```python
from build123d import *


with BuildPart() as f2:
    # F2: sweep along a path in F1
    with BuildLine(Plane.XY) as f2_path:
        Line((0, 0), (0, 50.8))
        ThreePointArc((0, 50.8), (-20.17757, 70.97757), (-40.35514, 50.8))
    # F0 (on Front) → F2 (sweep)
    with BuildSketch(Plane.XZ):
        Polygon((11.046861, 1.856294), (7.269184, 8.522789), (0.090175, 11.201377), (-7.131028, 8.638716), (-11.015544, 2.033904), (-9.745764, -5.522594), (-3.915833, -10.495009), (3.74636, -10.556693), (9.655589, -5.678782), align=None)
    sweep(path=f2_path.line)


solid = f2.part
```
Check sheet for the modelled part. Datum: model origin and axes. Units: mm. A direction names the side the tool comes from. Give positions to 0.01 mm unless a question says otherwise; leave off trailing zeros. Order: outer loops, then holes, each group sorted by start corner. A loop starts at its lowest first (then second) coordinate and runs counter-clockwise, first axis right, second up. Notation, with made-up numbers: (1, 12.5) -> (23, 12.5) arc R19 ccw to (23, 26.5) -> close; hole circle Ø8 at (50, 1.25). An arc over 180 degrees is marked (long way). Use CSV: the item, a comma, the result in double quotes. Start each with the question number.
1) Sectioned sample at C-C, the plane z = -2.75. Record the boundary of the cut face in (x, y).
2) Set-up check for faces 4 (the face through (-19.64, 75.09, -10.25)), 5 (the face through (-9.046, 25.756, 5.383)), 6 (the face through (9.184, 25.756, 5.143)), 7 (the face through (-41, 50.8, 0)), 8 (the face through (-6.872, 25.756, -7.974)): record each of +Z, -Z, +X, -X, +Y, -Y from which the full face is reachable in a straight line by a thin tool's end or side.
3) Material ranges on line 1 (X direction, y = 55, z = -1.25); line 2 (X direction, y = 53, z = 7); line 3 (Y direction, x = -11, z = 8), recorded low to high. Write a range as from..to.
4) Go/stop test with flat-tipped pins: P1, Ø10, axis at x = -6, y = 32, coming from the -Z side; P2, Ø2, axis at x = -4.5, y = 14, coming from the +Z side; P3, Ø2, axis at x = -28, z = -0.5, coming from the -Y side. Record where each tip stops, or that it passes through.
5) Mould release check, pull along X, two halves, no side actions. Record for faces 1 (the face through (-19.94, 61.59, -5.83)), 2 (the face through (3.73, 25.756, 9.843)), 3 (the face through (-3.47, 25.76, 9.94)): released by +X, released by -X, zero draft, split by the parting line, or undercut.
6) Sectioned sample at A-A, the plane y = 32.5. Record the boundary of the cut face in (x, z) (3 decimals), plus the area to 3 significant figures.
Recorded:
1,outline,"(-50.55, 50.8) -> (-30.14, 50.8) arc R9.97 cw to (-10.21, 50.8) -> (-10.21, 0) -> (10.2, 0) -> (10.2, 50.8) arc R30.37 ccw to start"
2,face 4,"-Z, +Y"
2,face 5,"+Z, -X, -Y"
2,face 6,"+Z, +X, +Y, -Y"
2,face 7,"+Z, -Z, -X, -Y"
2,face 8,"-Z, -X, -Y"
3,line 1,"-50.54..-28.94, -11.42..10.18"
3,line 2,"-48.4..-32.06, -8.3..8.05"
3,line 3,"59.54..76.98"
4,P1,"z = -10.52"
4,P2,"z = 9.93"
4,P3,"y = 54.51"
5,face 1,"undercut"
5,face 2,"released by +X"
5,face 3,"released by -X"
6,outline,"(-11.016, 2.034) -> (-9.746, -5.523) -> (-3.916, -10.495) -> (3.746, -10.557) -> (9.656, -5.679) -> (11.047, 1.856) -> (7.269, 8.523) -> (0.09, 11.201) -> (-7.131, 8.639) -> close"
6,area,"363 mm2"
